```python
from build123d import *

# Parameters (mm, degrees)
F0_W     = 100
F0_H     = 100
F1_DEPTH = 2
F2_R     = 15
F3_DEPTH = 25
F4_W     = 100
F4_H     = 50
F5_DEPTH = 2
F6_R     = 5


with BuildPart() as f1:
    # F0 (on Front) → F1 (new body)
    with BuildSketch(Plane.XZ):
        Rectangle(F0_W, F0_H)
    extrude(amount=F1_DEPTH)

    # F2 (on face) → F3 (cut)
    with BuildSketch(Plane.XZ.offset(2)):
        Circle(F2_R)
    extrude(amount=-F3_DEPTH, mode=Mode.SUBTRACT)

    # F4 (on face) → F5 (join)
    with BuildSketch(Plane(origin=(0, 0, -50), x_dir=(1, 0, 0), z_dir=(0, 0, -1))):
        with Locations((0, -25)):
            Rectangle(F4_W, F4_H)
    extrude(amount=-F5_DEPTH)

    # F6
    f6_edges = [f1.edges().sort_by_distance(p)[0] for p in [
        (50, -1, 50),
        (50, 50, -49),
        (-50, 50, -49),
        (-50, -1, 50),
    ]]
    fillet(f6_edges, radius=F6_R)


solid = f1.part
```
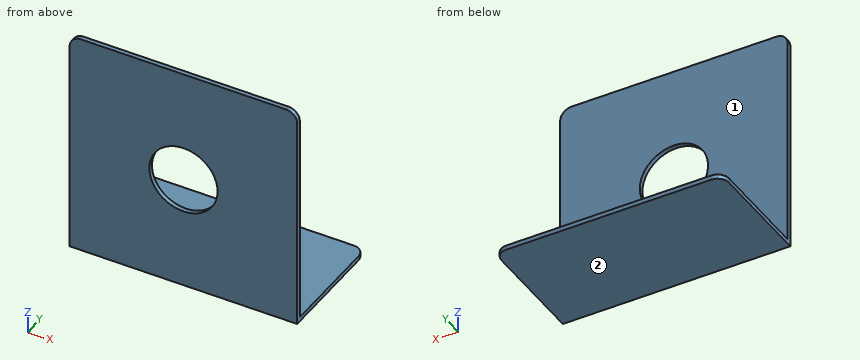
Could you check a few things on this model? Use its own coordinates, in mm. Face numbers are marked on the shaded views. A direction names the side the tool comes from. Coordinates: 2 decimals unless noted, no trailing zeros. Write each loop counter-clockwise with the first axis right and the second up, starting at its lowest first coordinate (ties: lowest second). Pieces come first, ordered by that corner, then holes. Notation, with made-up numbers: (-17.5, -1.75) -> (18.5, -1.75) arc R19 cw to (18.5, 7.25) -> close; hole circle Ø4 at (19.5, 36). An arc over 180 degrees is marked (long way). One line per question, with ' | ' between items. Start each with the question number.
1. If we section it at B-B (x = 0): Please give me the cut outline in (y, z), and give its area (3 significant figures).
2. If we section it at D-D (z = -16.5): Please give me the cut outline in (x, y), and give its area (3 significant figures).
3. Please list where these lines run through material, in increasing order: line 1 along Z through (x, y) = (0, -1.5); line 2 along Y through (x, z) = (-43, -10); line 3 along Z through (x, y) = (29.5, 6.5).
4. If we section it at C-C (x = -22): Please give me the cut outline in (y, z), and give its area (3 significant figures).
5. For the marked faces 1 and 2, which set-ups out of +Z, -Z, +X, -X, +Y, -Y let a thin tool reach every point of the face, with its end or its side?
6. If we section it at A-A (z = 0): Please give me the cut outline in (x, y), and give its area (3 significant figures).
7. Will this pin go through, and if not, where does the flat tip stop? P1, Ø2, axis at x = 24.5, y = 36, coming from the +Z side.
Return value:
1) outline: (-2, -50) -> (50, -50) -> (50, -48) -> (0, -48) -> (0, -15) -> (-2, -15) -> close; (-2, 15) -> (0, 15) -> (0, 50) -> (-2, 50) -> close | area: 240 mm²
2) outline: (-50, -2) -> (50, -2) -> (50, 0) -> (-50, 0) -> close | area: 200 mm²
3) line 1: z = -50 to -15, 15 to 50 | line 2: y = -2 to 0 | line 3: z = -50 to -48
4) outline: (-2, -50) -> (50, -50) -> (50, -48) -> (0, -48) -> (0, 50) -> (-2, 50) -> close | area: 300 mm²
5) face 1: +Z, +X, -X, +Y | face 2: -Z, +X, -X, +Y, -Y
6) outline: (-50, -2) -> (-15, -2) -> (-15, 0) -> (-50, 0) -> close; (15, -2) -> (50, -2) -> (50, 0) -> (15, 0) -> close | area: 140 mm²
7) P1: stops at z = -48
